The listing builds one solid part. Answer for the finished solid, in the listing's coordinates (mm). A direction names the side the tool comes from. Round coordinates to 2 decimals unless told otherwise and drop trailing zeros. Write each loop counter-clockwise with the first axis right and the second up, starting at its lowest first coordinate (ties: lowest second). Pieces come first, ordered by that corner, then holes.
Item 1: Each of these flat-tipped pins is pushed along its axis until it touches: pin 1 (4 mm diameter, centred on x = -14, y = -36, fed in from -Z); pin 2 (4 mm diameter, centred on x = -13, y = -50, fed in from +Z). Where does it stop, or does it pass through?
Item 2: For a pull along Z with two mould halves and no side action, classify faces 1 (the face through (-8, -76.2, 64)), 2 (the face through (-8.543, -38, 92)), 3 (the face through (-8.121, -1.528, 1.449)) as +Z half, -Z half, draft (parallel to the pull), parting line (faces both ways), or undercut.
Item 3: Find the intervals of material crossed by probe 1 along Z at (x, y) = (-10.25, -37); probe 2 along Z at (x, y) = (-12.75, -12); probe 3 along X at (y, z) = (-31.5, 94.5), in increasing order.
Item 4: Find section D-D on z = 20.5. Give the vertices of the cut face in (x, y).
Item 5: Find section B-B on y = -54. Give the vertices of the cut face in (x, z), then the cut area to 3 significant figures.
Item 6: Find section C-C on z = 85. Give the vertices of the cut face in (x, y), then the cut area to 3 significant figures.
Item 7: Find section A-A on x = -14.25. Give the vertices of the cut face in (y, z).
Item 8: A tool of negligible diameter and unlimited length cuts with its end or side. For faces 4 (the face through (-8.12, -74.67, 125.7)), 5 (the face through (-12, -38, 101.6)), from which of +Z, -Z, +X, -X, +Y, -Y can it reach the whole face along a straight path? Write none if from no direction.
```python
from build123d import *

# Parameters (mm, degrees)
F1_DEPTH     = 76.2
F2_R         = 5.08
F3_R         = 5.08
F4_T1_DEPTH  = 5.998990562
F4_S5_W      = 5.08
F4_S5_H      = 5.08
F4_T6_DEPTH  = 5.08
F4_S11_W     = 5.08
F4_S11_H     = 5.08
F4_T12_DEPTH = 5.08
F4_S17_W     = 5.08
F4_S17_H     = 5.08
F4_T18_DEPTH = 5.08
F4_S23_W     = 5.08
F4_S23_H     = 5.08
F4_T24_DEPTH = 5.08
F4_S29_W     = 5.08
F4_S29_H     = 5.08
F4_T30_DEPTH = 5.08
F4_S35_W     = 5.08
F4_S35_H     = 5.08
F4_T36_DEPTH = 5.08


# Not quite as in the source:
# - a fillet or chamfer that OpenCascade refuses, or shapes differently, is made with other operations: its cross-section is extruded or revolved along the edge and cut away or added


with BuildPart() as f1:
    # F0 (on Front) → F1 (new body)
    with BuildSketch(Plane.XZ):
        Polygon((-16.158990562, 0), (0, 0), (0, 127.1478682756), (-16.158990562, 127.1478682756), (-16.158990562, 101.6), (-8.5426843725, 101.6), (-8.5426843725, 82.55), (-16.158990562, 82.55), align=None)
    extrude(amount=F1_DEPTH)

    # F2
    f2_edges = [f1.edges().sort_by_distance(p)[0] for p in [
        (-8.079495, -76.2, 127.147868),
        (0, -38.1, 0),
        (0, -38.1, 127.147868),
        (0, 0, 63.573934),
        (0, -76.2, 63.573934),
    ]]
    fillet(f2_edges, radius=F2_R)

    # F3
    f3_edges = [f1.edges().sort_by_distance(p)[0] for p in [
        (-16.158991, -76.2, 41.275),
        (-16.158991, 0, 41.275),
        (-16.158991, -38.1, 0),
        (-16.158991, 0, 114.373934),
        (-16.158991, -35.56, 127.147868),
    ]]
    fillet(f3_edges, radius=F3_R)

    # F4: fillet of radius 5.08 on 3 edges, made by hand

    # F4_s2 → F4_t1 (cut)
    with BuildSketch(Plane.YZ.offset(-11.078990562)):
        with BuildLine():
            ThreePointArc((0, 122.0678682756), (-1.4878975516, 125.6599707241), (-5.08, 127.1478682756))
            Line((-5.08, 127.1478682756), (0, 127.1478682756))
            Line((0, 127.1478682756), (0, 122.0678682756))
        make_face()
        with BuildLine():
            ThreePointArc((-5.08, 0), (-1.4878975516, 1.4878975516), (0, 5.08))
            Line((0, 5.08), (0, 0))
            Line((0, 0), (-5.08, 0))
        make_face()
        with BuildLine():
            ThreePointArc((-71.12, 0), (-74.7121024484, 1.4878975516), (-76.2, 5.08))
            Line((-76.2, 5.08), (-76.2, 0))
            Line((-76.2, 0), (-71.12, 0))
        make_face()
    extrude(amount=F4_T1_DEPTH, mode=Mode.SUBTRACT)


with BuildPart() as f4_tool4:
    # F4_s5 → F4_t6 (new body)
    with BuildSketch(Plane.XY.offset(5.08)):
        with Locations((-13.618990562, -73.66)):
            Rectangle(F4_S5_W, F4_S5_H)
    extrude(amount=-F4_T6_DEPTH)

    # F4_s7 → F4_t8 (revolve, cut)
    with BuildSketch(Plane(origin=(-11.078990562, -71.12, 5.08), x_dir=(0.7071067812, 0.7071067812, 0), z_dir=(-0.7071067812, 0.7071067812, 0))):
        with BuildLine():
            ThreePointArc((0, -5.08), (5.08, 0), (0, 5.08))
            Line((0, 5.08), (0, -5.08))
        make_face()
    revolve(axis=Axis((-11.078990562, -71.12, 5.08), (0, 0, -1)), mode=Mode.SUBTRACT)


with BuildPart() as f1_1:
    add(f1.part)

    # F4_t3: cut F4_tool4
    add(f4_tool4.part, mode=Mode.SUBTRACT)


with BuildPart() as f4_tool10:
    # F4_s11 → F4_t12 (new body)
    with BuildSketch(Plane.XY.offset(5.08)):
        with Locations((-2.54, -73.66)):
            Rectangle(F4_S11_W, F4_S11_H)
    extrude(amount=-F4_T12_DEPTH)

    # F4_s13 → F4_t14 (revolve, cut)
    with BuildSketch(Plane(origin=(-5.08, -71.12, 5.08), x_dir=(-0.7071067812, 0.7071067812, 0), z_dir=(-0.7071067812, -0.7071067812, 0))):
        with BuildLine():
            ThreePointArc((0, -5.08), (5.08, 0), (0, 5.08))
            Line((0, 5.08), (0, -5.08))
        make_face()
    revolve(axis=Axis((-5.08, -71.12, 5.08), (0, 0, -1)), mode=Mode.SUBTRACT)


with BuildPart() as f1_2:
    add(f1_1.part)

    # F4_t9: cut F4_tool10
    add(f4_tool10.part, mode=Mode.SUBTRACT)


with BuildPart() as f4_tool16:
    # F4_s17 → F4_t18 (new body)
    with BuildSketch(Plane.XY.offset(5.08)):
        with Locations((-13.618990562, -2.54)):
            Rectangle(F4_S17_W, F4_S17_H)
    extrude(amount=-F4_T18_DEPTH)

    # F4_s19 → F4_t20 (revolve, cut)
    with BuildSketch(Plane(origin=(-11.078990562, -5.08, 5.08), x_dir=(0.7071067812, -0.7071067812, 0), z_dir=(0.7071067812, 0.7071067812, 0))):
        with BuildLine():
            ThreePointArc((0, -5.08), (5.08, 0), (0, 5.08))
            Line((0, 5.08), (0, -5.08))
        make_face()
    revolve(axis=Axis((-11.078990562, -5.08, 5.08), (0, 0, -1)), mode=Mode.SUBTRACT)


with BuildPart() as f1_3:
    add(f1_2.part)

    # F4_t15: cut F4_tool16
    add(f4_tool16.part, mode=Mode.SUBTRACT)


with BuildPart() as f4_tool22:
    # F4_s23 → F4_t24 (new body)
    with BuildSketch(Plane.XY.offset(5.08)):
        with Locations((-2.54, -2.54)):
            Rectangle(F4_S23_W, F4_S23_H)
    extrude(amount=-F4_T24_DEPTH)

    # F4_s25 → F4_t26 (revolve, cut)
    with BuildSketch(Plane(origin=(-5.08, -5.08, 5.08), x_dir=(-0.7071067812, -0.7071067812, 0), z_dir=(0.7071067812, -0.7071067812, 0))):
        with BuildLine():
            ThreePointArc((0, -5.08), (5.08, 0), (0, 5.08))
            Line((0, 5.08), (0, -5.08))
        make_face()
    revolve(axis=Axis((-5.08, -5.08, 5.08), (0, 0, -1)), mode=Mode.SUBTRACT)


with BuildPart() as f1_4:
    add(f1_3.part)

    # F4_t21: cut F4_tool22
    add(f4_tool22.part, mode=Mode.SUBTRACT)


with BuildPart() as f4_tool28:
    # F4_s29 → F4_t30 (new body)
    with BuildSketch(Plane.XZ.offset(5.08)):
        with Locations((-2.54, 124.6078682756)):
            Rectangle(F4_S29_W, F4_S29_H)
    extrude(amount=-F4_T30_DEPTH)

    # F4_s31 → F4_t32 (revolve, cut)
    with BuildSketch(Plane(origin=(-5.08, -5.08, 122.0678682756), x_dir=(-0.7071067812, 0, -0.7071067812), z_dir=(0.7071067812, 0, -0.7071067812))):
        with BuildLine():
            ThreePointArc((0, -5.08), (5.08, 0), (0, 5.08))
            Line((0, 5.08), (0, -5.08))
        make_face()
    revolve(axis=Axis((-5.08, -5.08, 122.0678682756), (0, 1, 0)), mode=Mode.SUBTRACT)


with BuildPart() as f1_5:
    add(f1_4.part)

    # F4_t27: cut F4_tool28
    add(f4_tool28.part, mode=Mode.SUBTRACT)


with BuildPart() as f4_tool34:
    # F4_s35 → F4_t36 (new body)
    with BuildSketch(Plane.XZ.offset(5.08)):
        with Locations((-13.618990562, 124.6078682756)):
            Rectangle(F4_S35_W, F4_S35_H)
    extrude(amount=-F4_T36_DEPTH)

    # F4_s37 → F4_t38 (revolve, cut)
    with BuildSketch(Plane(origin=(-11.078990562, -5.08, 122.0678682756), x_dir=(0.7071067812, 0, -0.7071067812), z_dir=(0.7071067812, 0, 0.7071067812))):
        with BuildLine():
            ThreePointArc((0, -5.08), (5.08, 0), (0, 5.08))
            Line((0, 5.08), (0, -5.08))
        make_face()
    revolve(axis=Axis((-11.078990562, -5.08, 122.0678682756), (0, 1, 0)), mode=Mode.SUBTRACT)


with BuildPart() as f1_6:
    add(f1_5.part)

    # F4_t33: cut F4_tool34
    add(f4_tool34.part, mode=Mode.SUBTRACT)


solid = f1_6.part
```
Check values:
1. pin 1: stops at z = 0.08
1. pin 2: stops at z = 127.15
2. face 1: draft
2. face 2: undercut
2. face 3: -Z half
3. probe 1: z = 0 to 82.55, 101.6 to 127.15
3. probe 2: z = 0.28 to 82.55, 101.6 to 126.87
3. probe 3: x = -8.54 to 0
4. outline: (-16.16, -71.12) arc R5.08 ccw to (-11.08, -76.2) - (-5.08, -76.2) arc R5.08 ccw to (0, -71.12) - (0, -5.08) arc R5.08 ccw to (-5.08, 0) - (-11.08, 0) arc R5.08 ccw to (-16.16, -5.08) - close
5. outline: (-16.16, 5.08) arc R5.08 ccw to (-11.08, 0) - (-5.08, 0) arc R5.08 ccw to (0, 5.08) - (0, 122.07) arc R5.08 ccw to (-5.08, 127.15) - (-11.08, 127.15) arc R5.08 ccw to (-16.16, 122.07) - (-16.16, 101.6) - (-8.54, 101.6) - (-8.54, 82.55) - (-16.16, 82.55) - close
5. area: 1,890 mm2
6. outline: (-8.54, -76.2) - (-5.08, -76.2) arc R5.08 ccw to (0, -71.12) - (0, -5.08) arc R5.08 ccw to (-5.08, 0) - (-8.54, 0) - close
6. area: 640 mm2
7. outline: (-75.09, 5.08) arc R3.97 ccw to (-71.12, 1.11) - (-5.08, 1.11) arc R3.97 ccw to (-1.11, 5.08) - (-1.11, 82.55) - (-75.09, 82.55) - close; (-75.09, 101.6) - (-1.11, 101.6) - (-1.11, 122.07) arc R3.97 ccw to (-5.08, 126.04) - (-71.12, 126.04) arc R3.97 ccw to (-75.09, 122.07) - close
8. face 4: +Z, +X, -X, -Y
8. face 5: -X, +Y, -Y
